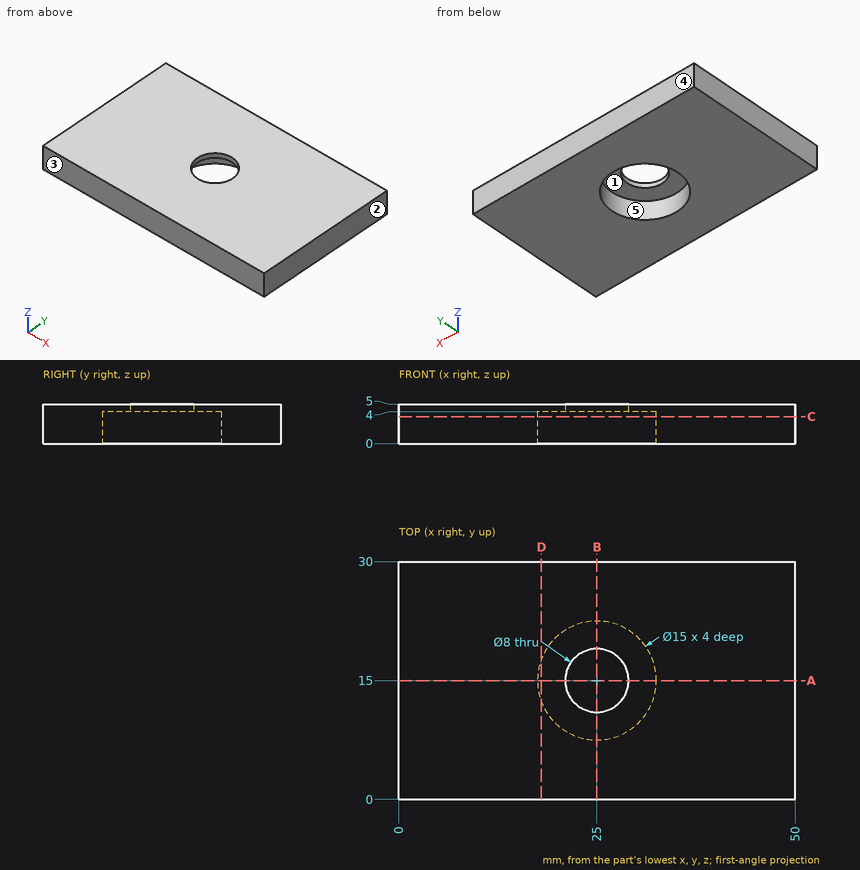
Geometry check sheet. Reference: drawing and pictorial views, mm from the part's lowest x, y, z. A direction names the side the tool comes from. Round coordinates to 2 decimals unless told otherwise and drop trailing zeros. Loops run counter-clockwise (first coordinate to the right, second up) from the corner with the lowest first, then second, coordinate; pieces in that order, holes last. Notation, with made-up numbers: M 32,69 L 55,69 A28 ccw 55,94 Z; hole C -4.75,17.5 d2. An arc over 180 degrees is marked long. Return JSON: item names as keys, results as strings. Group by question number.
(1) Mould release check, pull along Y, two halves, no side actions. Record for the marked faces 1, 2 and 3: pulls with the +Y half, pulls with the -Y half, needs draft (parallel to the pull), parting line crosses it, or undercut.
(2) Section check A-A, the plane y = 15. Enter the section's corners in (x, z).
(3) Go/stop test with a flat-tipped pin: pin 1 (13 mm diameter, centred on x = 25, y = 15, fed in from -Z). Record where the tip stops, or that it passes through.
(4) Section check B-B, the plane x = 25. Enter the section's corners in (y, z), and give its area (3 significant figures).
(5) Section check D-D, the plane x = 18. Enter the section's corners in (y, z).
(6) Section check C-C, the plane z = 3.4. Enter the section's corners in (x, y).
(7) Set-up check for the marked faces 4 and 5: record each of +Z, -Z, +X, -X, +Y, -Y from which the full face is reachable in a straight line by a thin tool's end or side.
(8) Scan lines: line 1 along Y through (x, z) = (25, 1); line 2 along Y through (x, z) = (23, 1.85); line 3 along X through (y, z) = (18.75, 3.5). Record each from-to range of solid material in increasing order. Write a range as [from, to].
Data:
{
 "1": {"face 1": "undercut", "face 2": "needs draft", "face 3": "pulls with the -Y half"},
 "2": {"outline": "M 0,0 L 17.5,0 L 17.5,4 L 21,4 L 21,5 L 0,5 Z; M 29,4 L 32.5,4 L 32.5,0 L 50,0 L 50,5 L 29,5 Z"},
 "3": {"pin 1": "z = 4"},
 "4": {"outline": "M 0,0 L 7.5,0 L 7.5,4 L 11,4 L 11,5 L 0,5 Z; M 19,4 L 22.5,4 L 22.5,0 L 30,0 L 30,5 L 19,5 Z", "area": "82.0 mm²"},
 "5": {"outline": "M 0,0 L 12.31,0 L 12.31,4 L 17.69,4 L 17.69,0 L 30,0 L 30,5 L 0,5 Z"},
 "6": {"outline": "M 0,0 L 50,0 L 50,30 L 0,30 Z; hole C 25,15 d15"},
 "7": {"face 4": "+Z, -Z, +X, -X, +Y", "face 5": "-Z"},
 "8": {"line 1": "[0, 7.5], [22.5, 30]", "line 2": "[0, 7.77], [22.23, 30]", "line 3": "[0, 18.5], [31.5, 50]"}
}
